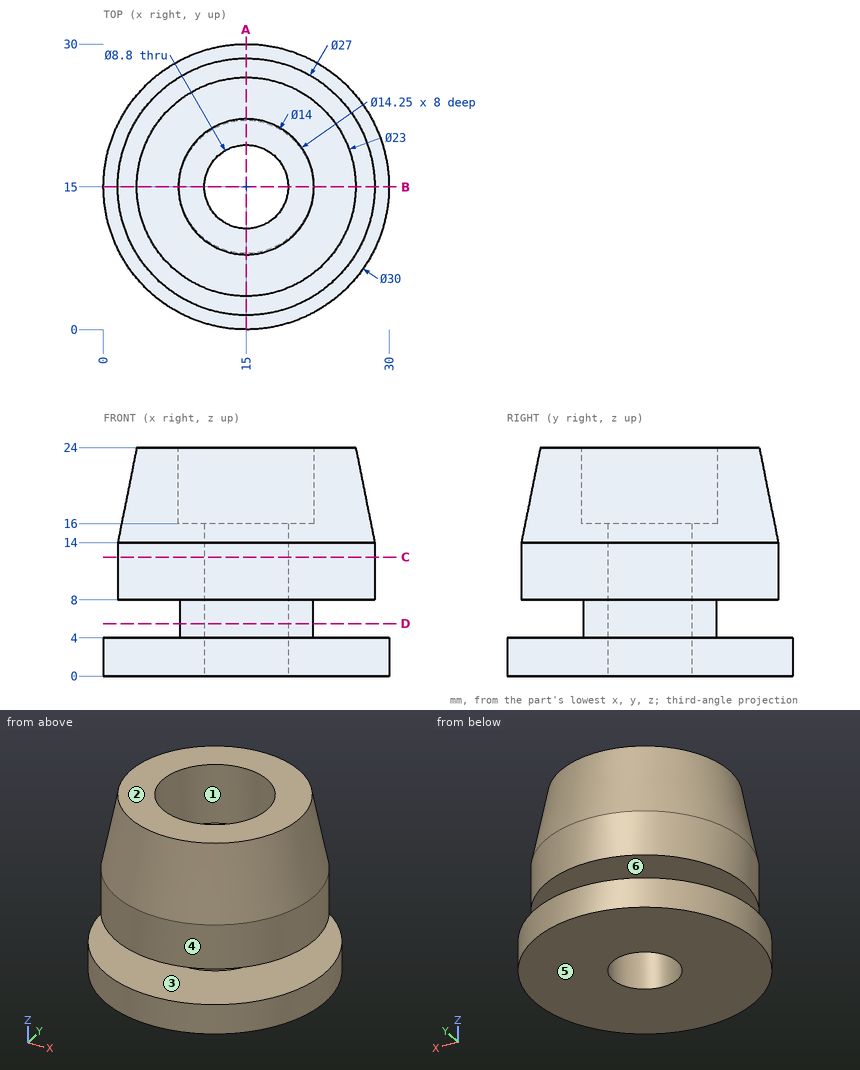
Geometry check sheet. Reference: drawing and pictorial views, mm from the part's lowest x, y, z. A direction names the side the tool comes from. Give positions to 0.01 mm unless a question says otherwise; leave off trailing zeros. Order: outer loops, then holes, each group sorted by start corner. A loop starts at its lowest first (then second) coordinate and runs counter-clockwise, first axis right, second up. Notation, with made-up numbers: M 53,45.25 L 78,45.25 A15 ccw 78,61.25 Z; hole C 30,10 d5. An arc over 180 degrees is marked long. Answer in a Markdown table with one row per item.
1) Thickness scan on L1, parallel to Y at x = 15, z = 5; L2, parallel to Z at x = 8.5, y = 1.75; L3, parallel to Z at x = 18.5, y = 6.25. Record the ranges inside material, lowest first. Write a range as [from, to].
Filled sheet:
| item | result |
|---|---|
| L1 | y = [8, 10.6], [19.4, 22] |
| L2 | z = [0, 4] |
| L3 | z = [0, 4], [8, 24] |
2) Access from +Z, -Z, +X, -X, +Y, -Y to the whole of each face (thin tool, end or side, straight path). Record for the marked faces 1, 2 and 3.
Filled sheet:
| item | result |
|---|---|
| face 1 | +Z |
| face 2 | +Z, +X, -X, +Y, -Y |
| face 3 | none |
3) Gauge pin test, flat ends, axial feed: P1, Ø1.5, axis at x = 17, z = 19, coming from the -Y side; P2, Ø3, axis at y = 6, z = 17.5, coming from the -X side; P3, Ø4, axis at x = 23.5, z = 17, coming from the -Y side. Record the tip position at first contact, or that the pin passes through.
Filled sheet:
| item | result |
|---|---|
| P1 | stops at y = 2.47 |
| P2 | stops at x = 4.57 |
| P3 | stops at y = 3.77 |
4) Cross-section at D-D, the plane z = 5.5. Enter the section's corners in (x, y), plus the area to 3 significant figures.
Filled sheet:
| item | result |
|---|---|
| outline | C 15,15 d14; hole C 15,15 d8.8 |
| area | 93.1 mm2 |
5) Cross-section at A-A, the plane x = 15. Enter the section's corners in (y, z) (3 decimals), plus the area to 3 significant figures.
Filled sheet:
| item | result |
|---|---|
| outline | M 0,0 L 10.6,0 L 10.6,16 L 7.875,16 L 7.875,24 L 3.5,24 L 1.5,14 L 1.5,8 L 8,8 L 8,4 L 0,4 Z; M 19.4,0 L 30,0 L 30,4 L 22,4 L 22,8 L 28.5,8 L 28.5,14 L 26.5,24 L 22.125,24 L 22.125,16 L 19.4,16 Z |
| area | 333 mm2 |
6) Cross-section at C-C, the plane z = 12.5. Enter the section's corners in (x, y), plus the area to 3 significant figures.
Filled sheet:
| item | result |
|---|---|
| outline | C 15,15 d27; hole C 15,15 d8.8 |
| area | 512 mm2 |
7) Release check for a two-part mould opening along Z. For the marked faces 4, 5 and 6 record: +Z half, -Z half, draft (parallel to the pull), parting line (faces both ways), or undercut.
Filled sheet:
| item | result |
|---|---|
| face 4 | draft |
| face 5 | -Z half |
| face 6 | undercut |
